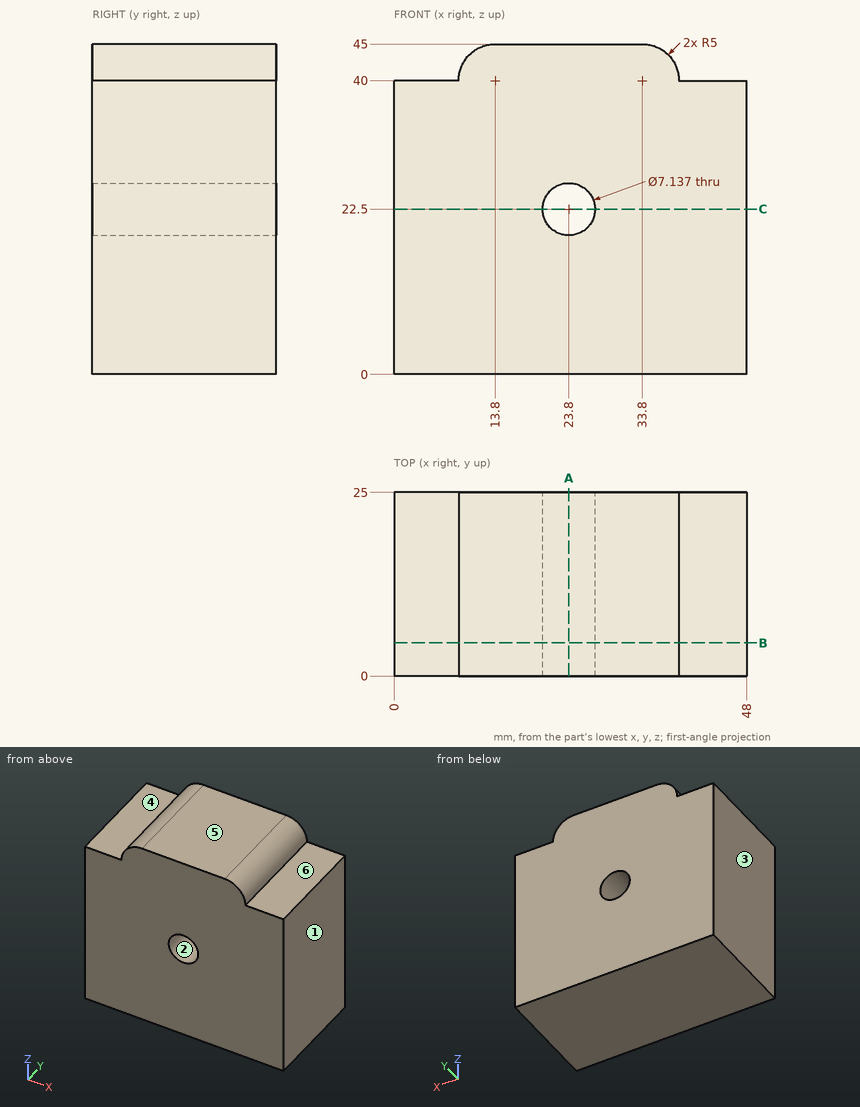
Source: three-view drawing plus pictorial views. Frame: mm from the lowest corner of the part. A direction names the side the tool comes from. Coordinates: 2 decimals unless noted, no trailing zeros. Order: outer loops, then holes, each group sorted by start corner. A loop starts at its lowest first (then second) coordinate and runs counter-clockwise, first axis right, second up.
Item 1: Material intervals for line 1 (Z direction, x = 23.8, y = 11); line 2 (Z direction, x = 42, y = 20.5); line 3 (X direction, y = 14.5, z = 20.5) (1 decimal), sorted ascending.
Output values:
line 1: z = 0 to 18.93, 26.07 to 45
line 2: z = 0 to 40
line 3: x = 0 to 20.8, 26.8 to 48
Item 2: Pull-direction query (X, two-part tool) for the marked faces 1, 2, 3 and 4; classes: pulls with the +X half, pulls with the -X half, needs draft (parallel to the pull), parting line crosses it, or undercut.
Output values:
face 1: pulls with the +X half
face 2: undercut
face 3: pulls with the -X half
face 4: needs draft
Item 3: Cut plane C-C (z = 22.5). Return loops of the section in (x, y), plus the area to 3 significant figures.
Output values:
outline: (0, 0) - (20.23, 0) - (20.23, 25) - (0, 25) - close; (27.37, 0) - (48, 0) - (48, 25) - (27.37, 25) - close
area: 1,020 mm2
Item 4: Cut plane A-A (x = 23.8). Return loops of the section in (y, z).
Output values:
outline: (0, 0) - (25, 0) - (25, 18.93) - (0, 18.93) - close; (0, 26.07) - (25, 26.07) - (25, 45) - (0, 45) - close
Item 5: First-contact query: P1, Ø7.5, axis at x = 42, y = 18, coming from the +Z side; P2, Ø2, axis at x = 9, y = 18.5, coming from the +Z side; P3, Ø2.5, axis at x = 2.5, y = 17.5, coming from the +Z side. Flat tips, straight axial feed; report the tip coordinate or a pass-through.
Output values:
P1: stops at z = 42.28
P2: stops at z = 43.25
P3: stops at z = 40
Item 6: Set-up query: the marked faces 5 and 6. Return all of +Z, -Z, +X, -X, +Y, -Y with unobstructed straight access to the full face (end or side cutting, diameter ignored); none if empty.
Output values:
face 5: +Z, +X, -X, +Y, -Y
face 6: +Z, +X, +Y, -Y
Item 7: Cut plane B-B (y = 4.5). Return loops of the section in (x, z), plus the area to 3 significant figures.
Output values:
outline: (0, 0) - (48, 0) - (48, 40) - (38.8, 40) arc R5 ccw to (33.8, 45) - (13.8, 45) arc R5 ccw to (8.8, 40) - (0, 40) - close; hole circle Ø7.14 at (23.8, 22.5)
area: 2,020 mm2
